Here's the drawing with two shaded views (mm, measured from the low corner). I have some questions. Round coordinates to 2 decimals unless told otherwise and drop trailing zeros. Order: outer loops, then holes, each group sorted by start corner. A loop starts at its lowest first (then second) coordinate and runs counter-clockwise, first axis right, second up.
Q1. If we section it at A-A (y = 9.75): Please give me the cut outline in (x, z).
Q2. If I drill on line 1 (X direction, y = 6.5, z = 63.5), over which ranges is the centre line in solid material (lowest first)?
Q3. If we section it at D-D (x = 10.75): Please give me the cut outline in (y, z), plus the area to 3 significant figures.
Q4. Will these pins go through, and if not, where does the flat tip stop? P1, Ø0.8, axis at x = 29.5, z = 39, coming from the -Y side; P2, Ø12, axis at y = 12, z = 17.5, coming from the -X side; P3, Ø6.5, axis at x = 13.5, y = 3.5, coming from the +Z side; P4, Ø6, axis at x = 21, z = 5.5, coming from the +Y side.
Q5. We'd pull the mould along X, two halves only. Please class the marked faces 1, 2, 3 and 4: pulls with the +X half, pulls with the -X half, needs draft (parallel to the pull), parting line crosses it, or undercut.
Q6. If we section it at C-C (z = 18): Please give me the cut outline in (x, y), plus the area to 3 significant figures.
Q7. If we section it at B-B (z = 65): Please give me the cut outline in (x, y).
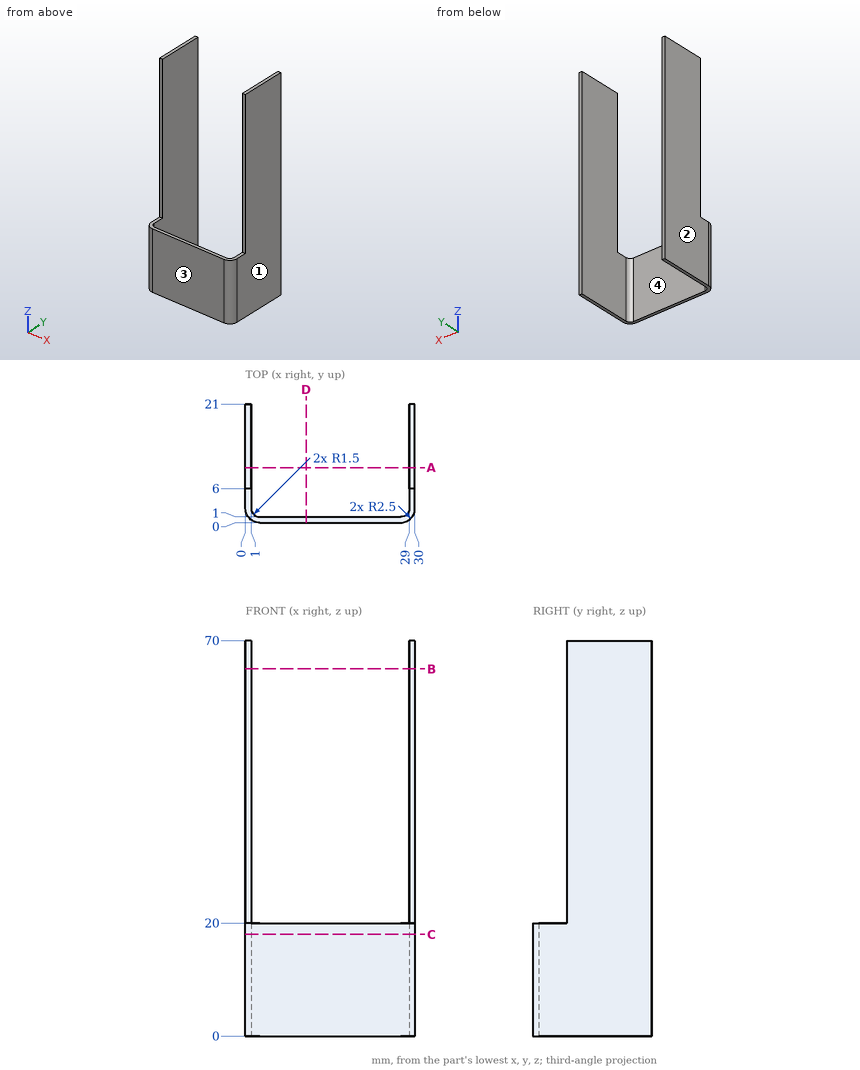
Solution:
1. outline: (0, 0) - (1, 0) - (1, 70) - (0, 70) - close; (29, 0) - (30, 0) - (30, 70) - (29, 70) - close
2. line 1: x = 0 to 1, 29 to 30
3. outline: (0, 0) - (1, 0) - (1, 20) - (0, 20) - close
3. area: 20.0 mm2
4. P1: stops at y = 6
4. P2: stops at x = 0
4. P3: stops at z = 20
4. P4: stops at y = 1
5. face 1: pulls with the +X half
5. face 2: pulls with the -X half
5. face 3: needs draft
5. face 4: undercut
6. outline: (0, 2.5) arc R2.5 ccw to (2.5, 0) - (27.5, 0) arc R2.5 ccw to (30, 2.5) - (30, 21) - (29, 21) - (29, 2.5) arc R1.5 cw to (27.5, 1) - (2.5, 1) arc R1.5 cw to (1, 2.5) - (1, 21) - (0, 21) - close
6. area: 68.3 mm2
7. outline: (0, 6) - (1, 6) - (1, 21) - (0, 21) - close; (29, 6) - (30, 6) - (30, 21) - (29, 21) - close
